Build history of the part. All positions in model axes, mm. Round coordinates to 2 decimals unless told otherwise and drop trailing zeros. Loops run counter-clockwise (first coordinate to the right, second up) from the corner with the lowest first, then second, coordinate; pieces in that order, holes last. Notation, with made-up numbers: (27.25, 11.5) -> (55.25, 11.5) arc R17 ccw to (55.25, 23.5) -> close; hole circle Ø11 at (77.25, -38). An arc over 180 degrees is marked (long way). Put each result on its own line as item: value. Start each with the question number.
Item 1: Cut at A-A, the plane y = 0. List the corners of the cut face in (x, z), plus the area to 3 significant figures.
Item 2: Cut at C-C, the plane z = 1.25. List the corners of the cut face in (x, y), plus the area to 3 significant figures.
Item 3: Cut at B-B, the plane x = 27. List the corners of the cut face in (y, z).
Item 4: Cut at D-D, the plane x = -30.5. List the corners of the cut face in (y, z).
Item 5: Pull direction X, two halves, no side cores. Call faces 1 (the cylindrical face through (37.683, 3.364, 3.451)), 2 (the cylindrical face through (-39.434, -12.294, 3.479)), 3 (the cylindrical face through (39.434, -12.294, 3.479)): +X half, -X half, draft (parallel to the pull), parting line (faces both ways), or undercut.
Item 6: Drill centre lines: probe 1 along X at (y, z) = (0.5, 5); probe 2 along Y at (x, z) = (27, 4.75); probe 3 along X at (y, z) = (-2, 2.25). Where is each one in solid material? Low to high. Write a range as [from, to].
```python
from build123d import *

# Parameters (mm, degrees)
F0_R         = 11.2
F1_DEPTH     = 7
F2_R         = 2
F3_T1_DEPTH  = 7
F3_T4_ANGLE  = 90
F3_T6_ANGLE  = 90
F3_T8_ANGLE  = 90
F3_T10_ANGLE = 90
F3_T12_ANGLE = 90
F3_T14_ANGLE = 90
F3_T16_ANGLE = 90
F3_T18_ANGLE = 90


# Not quite as in the source:
# - a fillet or chamfer that OpenCascade refuses, or shapes differently, is made with other operations: its cross-section is extruded or revolved along the edge and cut away or added


with BuildPart() as f1:
    # F0 (on Top) → F1 (new body)
    with BuildSketch(Plane.XY):
        Polygon((42, 15), (0, 15), (-42, 15), (-42, -15), (42, -15), align=None)
        with Locations((-27, 0)):
            Circle(F0_R, mode=Mode.SUBTRACT)
        Circle(F0_R, mode=Mode.SUBTRACT)
        with Locations((27, 0)):
            Circle(F0_R, mode=Mode.SUBTRACT)
    extrude(amount=F1_DEPTH)

    # F2
    f2_edges = [f1.edges().sort_by_distance(p)[0] for p in [
        (0, 15, 7),
        (-42, 0, 7),
        (0, -15, 7),
        (42, 0, 7),
        (42, 0, 0),
        (0, 15, 0),
        (-42, 0, 0),
        (0, -15, 0),
    ]]
    fillet(f2_edges, radius=F2_R)

    # F3: fillet of radius 9 on 4 edges, made by hand

    # F3_s2 → F3_t1 (cut)
    with BuildSketch(Plane.XY):
        with BuildLine():
            ThreePointArc((-33, 15), (-39.3639610307, 12.3639610307), (-42, 6))
            Line((-42, 6), (-42, 15))
            Line((-42, 15), (-33, 15))
        make_face()
        with BuildLine():
            ThreePointArc((-42, -6), (-39.3639610307, -12.3639610307), (-33, -15))
            Line((-33, -15), (-42, -15))
            Line((-42, -15), (-42, -6))
        make_face()
        with BuildLine():
            ThreePointArc((42, -6), (39.3639610307, -12.3639610307), (33, -15))
            Line((33, -15), (42, -15))
            Line((42, -15), (42, -6))
        make_face()
        with BuildLine():
            ThreePointArc((33, 15), (39.3639610307, 12.3639610307), (42, 6))
            Line((42, 6), (42, 15))
            Line((42, 15), (33, 15))
        make_face()
    extrude(amount=F3_T1_DEPTH, mode=Mode.SUBTRACT)

    # F3_s3 → F3_t4 (revolve, cut)
    with BuildSketch(Plane.YZ.offset(33)):
        with BuildLine():
            ThreePointArc((13, 0), (14.4142135624, 0.5857864376), (15, 2))
            Line((15, 2), (15, 0))
            Line((15, 0), (13, 0))
        make_face()
    revolve(axis=Axis((33, 6, 0), (0, 0, -1)), revolution_arc=F3_T4_ANGLE, mode=Mode.SUBTRACT)

    # F3_s5 → F3_t6 (revolve, cut)
    with BuildSketch(Plane.XZ.offset(-6)):
        with BuildLine():
            ThreePointArc((40, 7), (41.4142135624, 6.4142135624), (42, 5))
            Line((42, 5), (42, 7))
            Line((42, 7), (40, 7))
        make_face()
    revolve(axis=Axis((33, 6, 7), (0, 0, 1)), revolution_arc=F3_T6_ANGLE, mode=Mode.SUBTRACT)

    # F3_s7 → F3_t8 (revolve, cut)
    with BuildSketch(Plane.XZ.offset(6)):
        with BuildLine():
            ThreePointArc((40, 0), (41.4142135624, 0.5857864376), (42, 2))
            Line((42, 2), (42, 0))
            Line((42, 0), (40, 0))
        make_face()
    revolve(axis=Axis((33, -6, 0), (0, 0, -1)), revolution_arc=F3_T8_ANGLE, mode=Mode.SUBTRACT)

    # F3_s9 → F3_t10 (revolve, cut)
    with BuildSketch(Plane.YZ.offset(33)):
        with BuildLine():
            ThreePointArc((-13, 7), (-14.4142135624, 6.4142135624), (-15, 5))
            Line((-15, 5), (-15, 7))
            Line((-15, 7), (-13, 7))
        make_face()
    revolve(axis=Axis((33, -6, 7), (0, 0, 1)), revolution_arc=F3_T10_ANGLE, mode=Mode.SUBTRACT)

    # F3_s11 → F3_t12 (revolve, cut)
    with BuildSketch(Plane.YZ.offset(-33)):
        with BuildLine():
            ThreePointArc((-13, 0), (-14.4142135624, 0.5857864376), (-15, 2))
            Line((-15, 2), (-15, 0))
            Line((-15, 0), (-13, 0))
        make_face()
    revolve(axis=Axis((-33, -6, 0), (0, 0, -1)), revolution_arc=F3_T12_ANGLE, mode=Mode.SUBTRACT)

    # F3_s13 → F3_t14 (revolve, cut)
    with BuildSketch(Plane.XZ.offset(6)):
        with BuildLine():
            ThreePointArc((-40, 7), (-41.4142135624, 6.4142135624), (-42, 5))
            Line((-42, 5), (-42, 7))
            Line((-42, 7), (-40, 7))
        make_face()
    revolve(axis=Axis((-33, -6, 7), (0, 0, 1)), revolution_arc=F3_T14_ANGLE, mode=Mode.SUBTRACT)

    # F3_s15 → F3_t16 (revolve, cut)
    with BuildSketch(Plane.XZ.offset(-6)):
        with BuildLine():
            ThreePointArc((-40, 0), (-41.4142135624, 0.5857864376), (-42, 2))
            Line((-42, 2), (-42, 0))
            Line((-42, 0), (-40, 0))
        make_face()
    revolve(axis=Axis((-33, 6, 0), (0, 0, -1)), revolution_arc=F3_T16_ANGLE, mode=Mode.SUBTRACT)

    # F3_s17 → F3_t18 (revolve, cut)
    with BuildSketch(Plane.YZ.offset(-33)):
        with BuildLine():
            ThreePointArc((13, 7), (14.4142135624, 6.4142135624), (15, 5))
            Line((15, 5), (15, 7))
            Line((15, 7), (13, 7))
        make_face()
    revolve(axis=Axis((-33, 6, 7), (0, 0, 1)), revolution_arc=F3_T18_ANGLE, mode=Mode.SUBTRACT)


solid = f1.part
```
Reply:
1. outline: (-42, 2) arc R2 ccw to (-40, 0) -> (-38.2, 0) -> (-38.2, 7) -> (-40, 7) arc R2 ccw to (-42, 5) -> close; (-15.8, 0) -> (-11.2, 0) -> (-11.2, 7) -> (-15.8, 7) -> close; (11.2, 0) -> (15.8, 0) -> (15.8, 7) -> (11.2, 7) -> close; (38.2, 0) -> (40, 0) arc R2 ccw to (42, 2) -> (42, 5) arc R2 ccw to (40, 7) -> (38.2, 7) -> close
1. area: 114 mm^2
2. outline: (-41.85, -6) arc R8.85 ccw to (-33, -14.85) -> (33, -14.85) arc R8.85 ccw to (41.85, -6) -> (41.85, 6) arc R8.85 ccw to (33, 14.85) -> (-33, 14.85) arc R8.85 ccw to (-41.85, 6) -> close; hole circle Ø22.4 at (-27, 0); hole circle Ø22.4 at (0, 0); hole circle Ø22.4 at (27, 0)
2. area: 1,240 mm^2
3. outline: (-15, 2) arc R2 ccw to (-13, 0) -> (-11.2, 0) -> (-11.2, 7) -> (-13, 7) arc R2 ccw to (-15, 5) -> close; (11.2, 0) -> (13, 0) arc R2 ccw to (15, 2) -> (15, 5) arc R2 ccw to (13, 7) -> (11.2, 7) -> close
4. outline: (-15, 2) arc R2 ccw to (-13, 0) -> (-10.64, 0) -> (-10.64, 7) -> (-13, 7) arc R2 ccw to (-15, 5) -> close; (10.64, 0) -> (13, 0) arc R2 ccw to (15, 2) -> (15, 5) arc R2 ccw to (13, 7) -> (10.64, 7) -> close
5. face 1: undercut
5. face 2: -X half
5. face 3: +X half
6. probe 1: x = [-42, -38.19], [-15.81, -11.19], [11.19, 15.81], [38.19, 42]
6. probe 2: y = [-15, -11.2], [11.2, 15]
6. probe 3: x = [-42, -38.02], [-15.98, -11.02], [11.02, 15.98], [38.02, 42]
